Source: CAD feature listing. Evaluate the final solid. Frame: model axes, mm. A direction names the side the tool comes from. Give positions to 0.01 mm unless a question says otherwise; leave off trailing zeros. Write each loop counter-clockwise with the first axis right and the second up, starting at its lowest first coordinate (ties: lowest second). Pieces come first, ordered by that corner, then holes. Notation, with made-up numbers: (8.25, 12) - (65.25, 12) arc R32 ccw to (65.25, 42) - close; hole circle Ø4 at (62.25, 12.25). An arc over 180 degrees is marked (long way). One line per question, with ' | ' between items. Start each with the question number.
(1) Ray query, line 1 (Z direction, x = -2, y = 6); line 2 (Y direction, x = 1.5, z = -4.75); line 3 (X direction, y = 24, z = 0). Return the intervals inside material, ascending. Write a range as [from, to].
(2) Pin query (flat end, axial travel): pin 1 (2.5 mm diameter, centred on x = -0.5, y = -2, fed in from +Z); pin 2 (4 mm diameter, centred on x = 3, y = 21.5, fed in from -Z); pin 3 (4 mm diameter, centred on x = 1.5, y = 10.5, fed in from -Z). Return the tip coordinate at first contact, or that it passes through.
(3) Access query for faces 4 (the flat face through (0, 0, 5)), 5 (the flat face through (-2.175, -2.873, -1.233)), 6 (the flat face through (-3, -4.4, 1)). Directions: +Z, -Z, +X, -X, +Y, -Y. A direction counts if a zero-diameter tool reaches every point of the face in a straight line with its end or side. Return the directions, or none.
(4) Draft query along Z for faces 1 (the flat face through (2.155, -2.873, -1.268)), 2 (the cylindrical face through (-0.867, 17.672, 3.905)), 3 (the flat face through (0, 35, 0)). Return one class per face: +Z half, -Z half, draft (parallel to the pull), parting line (faces both ways), or undercut.
(5) Section A-A, the plane y = 11.5. Return loops of the section in (x, z).
Solid Edge part; units mm, degrees
sketch "Sketch1" plane through (0, 0, 0) normal (0, 0, 1) x (1, 0, 0)
  line L0 (4, 0) -> (4, 35)
  line L1 (0, 35) -> (4, 35)
  line L2 (0, 0) -> (0, 35)
  line L3 (0, 0) -> (0, -4.4)
  line L4 (0, -4.4) -> (7, -4.4)
  line L5 (7, -4.4) -> (7, 0)
  line L6 (7, 0) -> (4, 0)
revolve "RevolvedProtrusion1" add sketch "Sketch1" angle 360 about axis through (0, 0, 0) along (0, 1, 0)
sketch "Sketch2" plane through (0, 0, 0) normal (1, 0, 0) x (0, 1, 0)
  line L0 (-4.4, 3.3615) -> (-1.8, 3.3615)
  line L1 (0.1408, 0) -> (-1.8, 3.3615)
  line L2 (-4.4, 0) -> (0.1408, 0)
  line L3 (-4.4, 0) -> (-4.4, 3.3615)
revolve "RevolvedCutout1" cut sketch "Sketch2" angle 360 about axis through (0, -4.5, 0) along (0, 1, 0)
sketch "Sketch3" plane through (0, -4.4, 0) normal (0, -1, 0) x (0, 0, 1)
  circle A0 centre (0, 0) radius 3.3615
  line L0 (-2.5, -1.4434) -> (0, -2.8868)
  line L1 (0, -2.8868) -> (2.5, -1.4434)
  line L2 (2.5, -1.4434) -> (2.5, 1.4434)
  line L3 (2.5, 1.4434) -> (0, 2.8868)
  line L4 (0, 2.8868) -> (-2.5, 1.4434)
  line L5 (-2.5, 1.4434) -> (-2.5, -1.4434)
extrude "Protrusion1" add sketch "Sketch3" against normal up to next
sketch "Sketch4" plane through (0, 0, 0) normal (0, 0, 1) x (1, 0, 0)
  line L0 (-2.8868, -4.4) -> (0, -4.4)
  line L1 (0, -4.4) -> (0, -3.6265)
  line L2 (0, -3.6265) -> (-2.8868, -4.4)
revolve "RevolvedCutout2" cut sketch "Sketch4" angle 360 about axis through (0, -4.5, 0) along (0, 1, 0)
fillet "Round1" radius 0.4 1 edges at (0, 0, -4)
chamfer "倒斜角_2" distance 0.5333 angle 45 1 edges at (0, 35, -4)
cosmetic_thread "螺纹_3" thread depth 32.5
sketch "Sketch5" plane through (0, 0, 0) normal (0, 0, 1) x (1, 0, 0)
  arc A0 (-3.8153, -4.4) -> (-7, 0) centre (-2.3681, 0) cw
revolve "RevolvedCutout3" cut sketch "Sketch5" angle 360 about axis through (0, 0, 0) along (0, -1, 0) material side at (-6.1609, -2.7452, 0)
Check sheet entries:
1) line 1: [-3.46, 3.46] | line 2: [-3.82, 0] | line 3: [-4, 4]
2) pin 1: z = 6.93 | pin 2: z = -3.87 | pin 3: z = -4
3) face 4: +Y | face 5: -Y | face 6: +Z, -Z, +X, -X, -Y
4) face 1: undercut | face 2: parting line | face 3: draft
5) outline: circle Ø8 at (0, 0)
